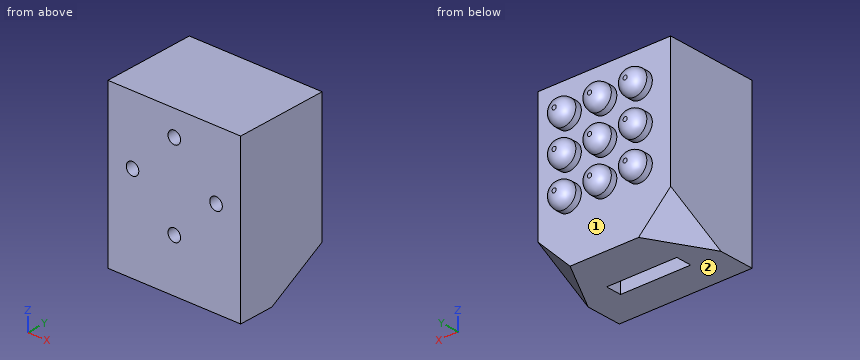
Autodesk Inventor part; units mm, degrees
ref_plane "Work Plane1" through (0, 22.2, -30.8) normal (-0.6571, -0.3693, 0.6571) x (-0.7071, 0, -0.7071)
ref_plane "Work Plane2" through (-15.9, 0, -38.5) normal (-1, 0, 0) x (0, 0, 1)
ref_plane "YZ Plane" through (0, 0, 0) normal (1, 0, 0) x (0, 1, 0)
sketch "Sketch1" plane through (0, 0, 0) normal (0, 1, 0) x (-1, 0, 0)
  line L0 (0, 0) -> (31.8, 0)
  line L1 (31.8, 0) -> (31.8, -38.5)
  line L2 (31.8, -38.5) -> (0, -38.5)
  line L3 (0, -38.5) -> (0, 0)
  dimension "d0" = 31.8
  dimension "d1" = 38.5
extrude "Extrusion1" add sketch "Sketch1" along normal blind 22.2
sketch "Sketch2" plane through (0, 0, 0) normal (0, -1, 0) x (1, 0, 0)
  line L0 (-31.8, 0) -> (0, 0)
  line L1 (-15.9, 0) -> (-15.9, -1.476)
  line L2 (-15.9, 0) -> (-15.9, -16)
  line L3 (-15.9, -16) -> (-5.9, -16)
  line L4 (-5.9, -16) -> (-25.9, -16)
  line L5 (-15.9, -16) -> (-15.9, -26)
  line L6 (-15.9, -26) -> (-15.9, -6)
  circle A0 centre (-15.9, -6) radius 1.5
  circle A1 centre (-5.9, -16) radius 1.5
  circle A2 centre (-15.9, -26) radius 1.5
  circle A3 centre (-25.9, -16) radius 1.5
  dimension "d4" = 16
  dimension "d5" = 10
  dimension "d6" = 20
  dimension "d7" = 10
  dimension "d8" = 20
  dimension "d9" = 3
  dimension "d10" = 3
  dimension "d11" = 3
  dimension "d12" = 3
extrude "Extrusion2" cut sketch "Sketch2" against normal blind 4.5
sketch "Sketch3" plane through (0, 22.2, 0) normal (0, 1, 0) x (1, 0, 0)
  line L0 (-31.8, 0) -> (0, 0)
  line L1 (-15.9, 0) -> (-15.9, 16)
  circle A0 centre (-15.9, 16) radius 3
  circle A1 centre (-7.4, 16) radius 3
  circle A2 centre (-24.4, 16) radius 3
  circle A3 centre (-7.4, 7.5) radius 3
  circle A4 centre (-15.9, 7.5) radius 3
  circle A5 centre (-24.4, 7.5) radius 3
  circle A6 centre (-7.4, 24.5) radius 3
  circle A7 centre (-15.9, 24.5) radius 3
  circle A8 centre (-24.4, 24.5) radius 3
  dimension "d15" = 16
  dimension "d16" = 6
  dimension "d19" = 8.5
  dimension "d26" = 8.5
  dimension "d33" = 8.5
  dimension "d40" = 8.5
extrude "Extrusion3" add sketch "Sketch3" along normal blind 4
fillet "Fillet1" radius 2.5 9 edges at (-10.4, 26.2, -7.5) (-18.9, 26.2, -7.5) (-27.4, 26.2, -7.5) (-27.4, 26.2, -16) (-18.9, 26.2, -16) (-10.4, 26.2, -16) (-10.4, 26.2, -24.5) (-18.9, 26.2, -24.5) (-27.4, 26.2, -24.5)
sketch "Sketch4" plane through (0, 0, -38.5) normal (0, 0, -1) x (-1, 0, 0)
  line L0 (17.4, 0) -> (14.4, 0)
  line L1 (15.9, 0) -> (15.9, 12)
  line L2 (15.9, 12) -> (24.3, 12)
  line L3 (15.9, 12) -> (24.3, 12) construction
  line L4 (24.3, 12) -> (7.5, 12)
  line L5 (7.5, 12) -> (7.5, 8.2)
  line L6 (7.5, 8.2) -> (24.3, 8.2)
  line L7 (24.3, 8.2) -> (24.3, 12)
  point P0 (0, 0)
  dimension "d48" = 12
  dimension "d49" = 8.4
  dimension "d50" = 0
  dimension "d51" = 16.8
  dimension "d52" = 3.8
extrude "Extrusion4" cut sketch "Sketch4" against normal blind 6
sketch3d "3D Sketch1"
ref_plane "Work Plane1" through (0, 22.2, -30.8) normal (-0.6571, -0.3693, 0.6571) x (-0.7071, 0, -0.7071)
sketch "Sketch5" plane through (0, 22.2, -30.8) normal (-0.6571, -0.3693, 0.6571) x (-0.7071, 0, -0.7071)
  line L0 (-21.7789, -8.0435) -> (5.4447, 2.0109)
  line L1 (-3.5227, -1.301) -> (16.1237, -1.301)
  line L2 (16.1237, -1.301) -> (16.1237, 19.91)
  line L3 (16.1237, 19.91) -> (-3.5227, 19.91)
  line L4 (-3.5227, 19.91) -> (-3.5227, -1.301)
  point P0 (-21.7789, 12.5869)
extrude "Extrusion5" cut sketch "Sketch5" against normal blind 6
ref_plane "Work Plane2" through (-15.9, 0, -38.5) normal (-1, 0, 0) x (0, 0, 1)
mirror "Mirror1" about plane through (-15.9, 0, -38.5) normal (-1, 0, 0) of "Extrusion5"
properties part number "Contactile Sensor"
For this review, take the finished solid that the model builds, in its own axes (mm). Face numbers are marked on the shaded views. A direction names the side the tool comes from. Give positions to 0.01 mm unless a question says otherwise; leave off trailing zeros. Write each loop counter-clockwise with the first axis right and the second up, starting at its lowest first coordinate (ties: lowest second). Pieces come first, ordered by that corner, then holes.
Item 1: Wall thickness on probe 1 along Z at (x, y) = (-15.9, 2.45); probe 2 along Z at (x, y) = (-25.9, 2.65); probe 3 along X at (y, z) = (2.4, -26): over which ranges is each line inside the solid? List them lowest first.
Item 2: Insertion check: P1, Ø2.5, axis at x = -25.9, z = -16, coming from the -Y side; P2, Ø1.1, axis at x = -16, y = 9, coming from the -Z side; P3, Ø1.8, axis at x = -17, z = -35, coming from the +Y side. Each pin has a flat end and moves straight along its axis. Give the tip position at first contact, or say it passes through.
Item 3: Take a section at C-C (z = -19.5). Give the boundary of the cut face in (x, y), and give its area (3 significant figures).
Item 4: Machinability: for the marked faces 1 and 2, which of the approach directions +Z, -Z, +X, -X, +Y, -Y give a long, thin tool a straight path to every point of the face, cutting with its end or side? Answer none if there is none.
Item 5: Take a section at B-B (y = 10.5). Give the boundary of the cut face in (x, z).
Item 6: Take a section at A-A (z = -34.5). Give the boundary of the cut face in (x, y), and give its area (3 significant figures).
Established:
1. probe 1: z = -38.5 to -27.5, -24.5 to -7.5, -4.5 to 0
1. probe 2: z = -38.5 to -17.5, -14.5 to 0
1. probe 3: x = -31.8 to -17.4, -14.4 to 0
2. P1: stops at y = 4.5
2. P2: stops at z = -32.5
2. P3: stops at y = 22.2
3. outline: (-31.8, 0) - (0, 0) - (0, 22.2) - (-31.8, 22.2) - close
3. area: 706 mm2
4. face 1: +Y
4. face 2: -Z, +X, -X, +Y, -Y
5. outline: (-31.8, -37.37) - (-30.67, -38.5) - (-24.3, -38.5) - (-24.3, -32.5) - (-7.5, -32.5) - (-7.5, -38.5) - (-1.13, -38.5) - (0, -37.37) - (0, 0) - (-31.8, 0) - close
6. outline: (-31.8, 0) - (0, 0) - (0, 15.61) - (-3.7, 22.2) - (-28.1, 22.2) - (-31.8, 15.61) - close; hole (-24.3, 8.2) - (-7.5, 8.2) - (-7.5, 12) - (-24.3, 12) - close
6. area: 618 mm2
